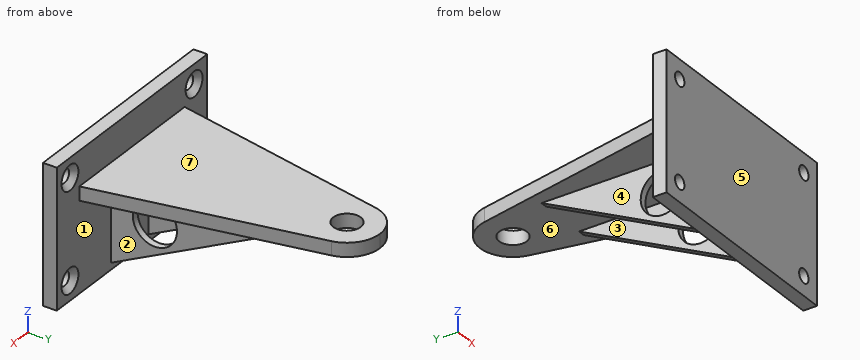
```python
from build123d import *

# Parameters (mm, degrees)
SKETCH2_W           = 80
SKETCH2_H           = 50
BOSS_EXTRUDE1_DEPTH = 5
BOSS_EXTRUDE2_DEPTH = 2.5
RIB1_REACH          = 112.227
SKETCH6_WALL_W      = 289.536116176
SKETCH6_WALL_H      = 2.5
SKETCH7_R           = 8
CUT_EXTRUDE1_DEPTH  = 2.5
SKETCH3_R           = 2.5
CUT_EXTRUDE2_DEPTH  = 5
CHAMFER1_SIZE       = 2
SKETCH8_R           = 5
CUT_EXTRUDE3_DEPTH  = 2.5


with BuildPart() as part:
    # Sketch2 → Boss-Extrude1 (new body)
    with BuildSketch(Plane(origin=(0, 0, 0), x_dir=(1, 0, 0), z_dir=(0, 1, 0))):
        Rectangle(SKETCH2_W, SKETCH2_H)
    extrude(amount=BOSS_EXTRUDE1_DEPTH)

    # Sketch4 → Boss-Extrude2 (add, symmetric)
    with BuildSketch(Plane.XY.offset(10)):
        with BuildLine():
            Line((0, 5), (-28, 5))
            Line((-28, 5), (-11.762376238, 85.376237624))
            ThreePointArc((-11.762376238, 85.376237624), (-7.598853483, 92.28748759), (0, 95))
            Line((0, 95), (0, 83))
            Line((0, 83), (0, 5))
        make_face()
    boss_extrude2 = extrude(amount=BOSS_EXTRUDE2_DEPTH, both=True)

    # Sketch6 wall → Rib1 (add, up to next)
    with BuildSketch(Plane(origin=(-10, 35, -7.5), x_dir=(0, -0.894427191, -0.4472135955), z_dir=(0, 0.4472135955, -0.894427191)), mode=Mode.PRIVATE) as rib1_sk1:
        Rectangle(SKETCH6_WALL_W, SKETCH6_WALL_H)
    rib1_tool1 = extrude(rib1_sk1.sketch, amount=-RIB1_REACH, mode=Mode.PRIVATE) - part.part
    rib1 = rib1_tool1.solids().sort_by_distance((-10, 35, -7.5))[0]
    add(rib1)

    # Sketch7 → Cut-Extrude1 (cut, symmetric)
    with BuildSketch(Plane(origin=(-10, 0, 0), x_dir=(0, 0, -1), z_dir=(1, 0, 0))):
        with Locations((3.5, 21)):
            Circle(SKETCH7_R)
    cut_extrude1 = extrude(amount=CUT_EXTRUDE1_DEPTH, both=True, mode=Mode.SUBTRACT)

    # Mirror2: Boss-Extrude2, Rib1, Cut-Extrude1 across plane
    add(boss_extrude2.mirror(Plane(origin=(0, 83, 7.5), x_dir=(0, 0, 1), z_dir=(1, 0, 0))))
    add(rib1.mirror(Plane(origin=(0, 83, 7.5), x_dir=(0, 0, 1), z_dir=(1, 0, 0))))
    add(cut_extrude1.mirror(Plane(origin=(0, 83, 7.5), x_dir=(0, 0, 1), z_dir=(1, 0, 0))), mode=Mode.SUBTRACT)

    # Sketch3 → Cut-Extrude2 (cut)
    with BuildSketch(Plane(origin=(0, 5, 0), x_dir=(1, 0, 0), z_dir=(0, 1, 0))):
        with Locations(Location((-33, 18, 0), (0, 0, 270))):
            Circle(SKETCH3_R)
        with Locations(Location((-33, -18, 0), (0, 0, 90))):
            Circle(SKETCH3_R)
        with Locations(Location((33, -18, 0), (0, 0, 270))):
            Circle(SKETCH3_R)
        with Locations(Location((33, 18, 0), (0, 0, 90))):
            Circle(SKETCH3_R)
    extrude(amount=-CUT_EXTRUDE2_DEPTH, mode=Mode.SUBTRACT)

    # Chamfer1
    chamfer1_edges = [part.edges().sort_by_distance(p)[0] for p in [
        (33, 5, -15.5),
        (33, 5, 15.5),
        (-33, 5, 20.5),
        (-33, 5, -20.5),
    ]]
    chamfer(chamfer1_edges, length=CHAMFER1_SIZE)

    # Sketch8 → Cut-Extrude3 (cut, symmetric)
    with BuildSketch(Plane.XY.offset(10)):
        with Locations((0, 83)):
            Circle(SKETCH8_R)
    extrude(amount=CUT_EXTRUDE3_DEPTH, both=True, mode=Mode.SUBTRACT)


solid = part.part
```
Can you work these out from the model? Positions are in its coordinate system, mm. Face numbers are marked on the shaded views. A direction names the side the tool comes from. Round coordinates to 2 decimals unless told otherwise and drop trailing zeros. Order: outer loops, then holes, each group sorted by start corner. A loop starts at its lowest first (then second) coordinate and runs counter-clockwise, first axis right, second up. Notation, with made-up numbers: (56.25, -39.5) -> (89.25, -39.5) arc R14 ccw to (89.25, -21.5) -> close; hole circle Ø7 at (-1, -14). An arc over 180 degrees is marked (long way). Return JSON: item names as keys, results as strings. Group by question number.
1. If we section it at C-C, the plane y = 21: Write out the boundary of the cut face in (x, z), then the cut area to 3 significant figures.
2. We'd pull the mould along X, two halves only. Please class the marked faces 1, 2, 3 and 4: released by +X, released by -X, zero draft, split by the parting line, or undercut.
3. If we section it at D-D, the plane y = 83: Write out the boundary of the cut face in (x, z), then the cut area to 3 significant figures.
4. If we section it at B-B, the plane x = 33: Write out the boundary of the cut face in (y, z).
5. Will these pins go through, and if not, where does the flat tip stop? pin 1 (1.5 mm diameter, centred on x = -17.5, y = 14, fed in from +Z); pin 2 (6 mm diameter, centred on x = -33, z = 18, fed in from -Y); pin 3 (15 mm diameter, centred on y = 27, z = -7, fed in from +X); pin 4 (1 mm diameter, centred on y = 60, z = 6, fed in from -X).
6. Which directions (+Z, -Z, +X, -X, +Y, -Y) give clear straight access to the entire face, cutting with the end or side of a thin tool? Please do the marked faces 5, 6 and 7.
7. If we section it at A-A, the plane z = -3.5: Write out the boundary of the cut face in (x, y).
8. I need wall thicknesses on line 1 (X direction, y = 1.2, z = -18); line 2 (X direction, y = 16, z = -12); line 3 (Y direction, x = -2.5, z = 20). Which ranges of each line are inside material? Lowest first, please. Write a range as [from, to].
Output values:
{
 "1": {"outline": "(-24.77, 7.5) -> (-11.25, 7.5) -> (-11.25, 4.5) -> (-8.75, 4.5) -> (-8.75, 7.5) -> (8.75, 7.5) -> (8.75, 4.5) -> (11.25, 4.5) -> (11.25, 7.5) -> (24.77, 7.5) -> (24.77, 12.5) -> (-24.77, 12.5) -> close; (-11.25, -14.5) -> (-8.75, -14.5) -> (-8.75, -11.5) -> (-11.25, -11.5) -> close; (8.75, -14.5) -> (11.25, -14.5) -> (11.25, -11.5) -> (8.75, -11.5) -> close", "area": "278 mm²"},
 "2": {"face 1": "undercut", "face 2": "released by +X", "face 3": "undercut", "face 4": "released by -X"},
 "3": {"outline": "(-12.24, 7.5) -> (-5, 7.5) -> (-5, 12.5) -> (-12.24, 12.5) -> close; (5, 7.5) -> (12.24, 7.5) -> (12.24, 12.5) -> (5, 12.5) -> close", "area": "72.4 mm²"},
 "4": {"outline": "(0, -25) -> (5, -25) -> (5, -22.5) -> (3, -20.5) -> (0, -20.5) -> close; (0, -15.5) -> (3, -15.5) -> (5, -13.5) -> (5, 13.5) -> (3, 15.5) -> (0, 15.5) -> close; (0, 20.5) -> (3, 20.5) -> (5, 22.5) -> (5, 25) -> (0, 25) -> close"},
 "5": {"pin 1": "z = 12.5", "pin 2": "y = 0", "pin 3": "x = 11.25", "pin 4": "x = -11.25"},
 "6": {"face 5": "+Z, -Z, +X, -X, -Y", "face 6": "-Z, +Y", "face 7": "+Z, +X, -X, +Y"},
 "7": {"outline": "(-40, 0) -> (40, 0) -> (40, 5) -> (11.25, 5) -> (11.25, 13) -> (8.75, 13) -> (8.75, 5) -> (-8.75, 5) -> (-8.75, 13) -> (-11.25, 13) -> (-11.25, 5) -> (-40, 5) -> close; (-11.25, 29) -> (-8.75, 29) -> (-8.75, 43) -> (-11.25, 43) -> close; (8.75, 29) -> (11.25, 29) -> (11.25, 43) -> (8.75, 43) -> close"},
 "8": {"line 1": "[-40, -35.5], [-30.5, 30.5], [35.5, 40]", "line 2": "[-11.25, -8.75], [8.75, 11.25]", "line 3": "[0, 5]"}
}
